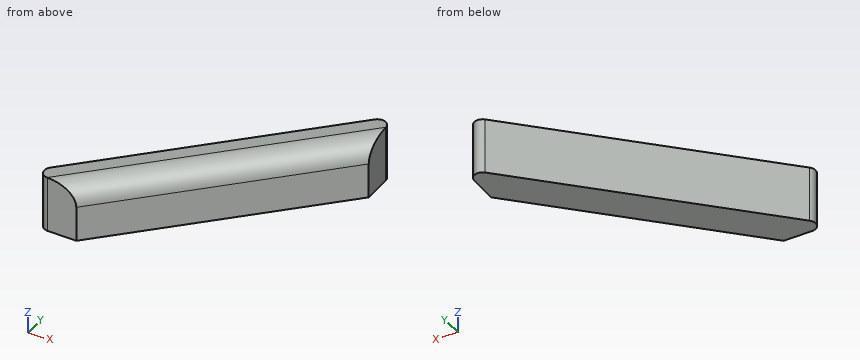
```python
from build123d import *

# Parameters (mm, degrees)
EXTRUDE_1_DEPTH = 13.5
FILLET_1_R      = 2
FILLET_2_R      = 2
FILLET_3_R      = 5


with BuildPart() as part:
    # 草图1 → 凸台-拉伸1 (new body)
    with BuildSketch(Plane.XY):
        Polygon((0, 0), (0, -11.7), (-44.194173824, -55.894173824), (-55.894173824, -55.894173824), align=None)
    extrude(amount=EXTRUDE_1_DEPTH)

    # 圆角1
    fillet_1_edges = [part.edges().sort_by_distance(p)[0] for p in [
        (-55.894173824, -55.894173824, 6.75),
    ]]
    fillet(fillet_1_edges, radius=FILLET_1_R)

    # 圆角2
    fillet_2_edges = [part.edges().sort_by_distance(p)[0] for p in [
        (0, 0, 6.75),
    ]]
    fillet(fillet_2_edges, radius=FILLET_2_R)

    # 圆角3
    fillet_3_edges = [part.edges().sort_by_distance(p)[0] for p in [
        (-22.097086912, -33.797086912, 13.5),
    ]]
    fillet(fillet_3_edges, radius=FILLET_3_R)


solid = part.part
```
Work out the finished part from the listing and answer in its coordinate system (mm). Give positions to 0.01 mm unless a question says otherwise; leave off trailing zeros. Loops run counter-clockwise (first coordinate to the right, second up) from the corner with the lowest first, then second, coordinate; pieces in that order, holes last. Notation, with made-up numbers: (-30, -23) -> (-12, -23) arc R30 cw to (-12, 4) -> close; hole circle Ø6 at (-9, 30.25). An arc over 180 degrees is marked (long way). Write item = value, one per line. Start each with the question number.
(1) Given pin 1 Ø4 at (y, z) = (-27.5, 8) entering from -X; pin 2 Ø2 at (x, z) = (-34.5, 9) entering from -Y; pin 3 Ø1.5 at (y, z) = (-26, 7) entering from -X; pin 4 Ø1 at (x, y) = (-44.5, -49) entering from -Z, each flat-ended and moving along its own axis, determine where each tip first touches the part or whether it passes through.
(2) Find section B-B on z = 10.5. Give the vertices of the cut face in (x, y).
(3) Find section A-A on z = 3.25. Give the vertices of the cut face in (x, y).
(4) Find the intervals of material crossed by probe 1 along X at (y, z) = (-47.5, 11); probe 2 along X at (y, z) = (-15, 7.75); probe 3 along Z at (x, y) = (-19.5, -27), in increasing order. Write a range as from..to.
From the geometry:
q1.pin_1 = -29.5
q1.pin_2 = -47.17
q1.pin_3 = -26.75
q1.pin_4 = 0
q2.outline = (-52.48, -52.48) arc R2 ccw to (-51.07, -55.89) -> (-44.78, -55.89) -> (0, -11.11) -> (0, -4.83) arc R2 ccw to (-3.41, -3.41) -> close
q3.outline = (-52.48, -52.48) arc R2 ccw to (-51.07, -55.89) -> (-44.19, -55.89) -> (0, -11.7) -> (0, -4.83) arc R2 ccw to (-3.41, -3.41) -> close
q4.probe_1 = -47.5..-36.75
q4.probe_2 = -15..-3.3
q4.probe_3 = 0..13.07
